For this review, take the finished solid that the model builds, in its own axes (mm). Round coordinates to 2 decimals unless told otherwise and drop trailing zeros. Loops run counter-clockwise (first coordinate to the right, second up) from the corner with the lowest first, then second, coordinate; pieces in that order, holes last. Notation, with made-up numbers: (59.5, 60.25) -> (64.5, 60.25) arc R27 ccw to (64.5, 76.25) -> close; hole circle Ø3 at (87, -17). An arc over 180 degrees is marked (long way). Write each question's results on one line, items separated by ' | '.
```python
from build123d import *

# Parameters (mm, degrees)
SKETCH1_R           = 2.35
BOSS_EXTRUDE1_DEPTH = 7.8


with BuildPart() as part:
    # Sketch1 → Boss-Extrude1 (new body)
    with BuildSketch(Plane(origin=(0, 0, 0), x_dir=(0, 0, -1), z_dir=(1, 0, 0))):
        with BuildLine():
            Line((-56, -3.73), (56, -3.73))
            ThreePointArc((56, -3.73), (59.73, 0), (56, 3.73))
            Line((56, 3.73), (-56, 3.73))
            ThreePointArc((-56, 3.73), (-59.73, 0), (-56, -3.73))
        make_face()
        with Locations((-56, 0)):
            Circle(SKETCH1_R, mode=Mode.SUBTRACT)
        with Locations((-48, 0)):
            Circle(SKETCH1_R, mode=Mode.SUBTRACT)
        with Locations((-40, 0)):
            Circle(SKETCH1_R, mode=Mode.SUBTRACT)
        with Locations((-32, 0)):
            Circle(SKETCH1_R, mode=Mode.SUBTRACT)
        with Locations((-24, 0)):
            Circle(SKETCH1_R, mode=Mode.SUBTRACT)
        with Locations((-16, 0)):
            Circle(SKETCH1_R, mode=Mode.SUBTRACT)
        with Locations((-8, 0)):
            Circle(SKETCH1_R, mode=Mode.SUBTRACT)
        Circle(SKETCH1_R, mode=Mode.SUBTRACT)
        with Locations((8, 0)):
            Circle(SKETCH1_R, mode=Mode.SUBTRACT)
        with Locations((16, 0)):
            Circle(SKETCH1_R, mode=Mode.SUBTRACT)
        with Locations((24, 0)):
            Circle(SKETCH1_R, mode=Mode.SUBTRACT)
        with Locations((32, 0)):
            Circle(SKETCH1_R, mode=Mode.SUBTRACT)
        with Locations((40, 0)):
            Circle(SKETCH1_R, mode=Mode.SUBTRACT)
        with Locations((48, 0)):
            Circle(SKETCH1_R, mode=Mode.SUBTRACT)
        with Locations((56, 0)):
            Circle(SKETCH1_R, mode=Mode.SUBTRACT)
    extrude(amount=BOSS_EXTRUDE1_DEPTH)


solid = part.part
```
1. To check wall thickness, follow probe 1 along Y at (x, z) = (5.5, -40); probe 2 along Y at (x, z) = (0.75, 30); probe 3 along Z at (x, y) = (7, 2.5). State the ranges of each line that lie inside material, in increasing order.
Values found:
probe 1: y = -3.73 to -2.35, 2.35 to 3.73 | probe 2: y = -3.73 to -1.23, 1.23 to 3.73 | probe 3: z = -58.77 to 58.77
2. Draft analysis for pull direction Z (two halves, no side actions). For faces 1 (the face through (3.845, 0.103, 18.348)), 2 (the face through (3.85, -0.08, -59.73)), 3 (the face through (4, 3.73, -1)), state which applies: released by +Z, released by -Z, zero draft, split by the parting line, or undercut.
Values found:
face 1: undercut | face 2: released by -Z | face 3: zero draft
3. For pin 1 (4 mm diameter, centred on y = 0, z = -8, fed in from -X); pin 2 (1.5 mm diameter, centred on y = 0.5, z = 11.5, fed in from -X), all flat-tipped, find the tip position at first contact; note any pin that passes through.
Values found:
pin 1: passes through | pin 2: stops at x = 0
4. Consider section A-A (z = -8). State the section outline as (x, y) points.
Values found:
outline: (0, -3.73) -> (7.8, -3.73) -> (7.8, -2.35) -> (0, -2.35) -> close; (0, 2.35) -> (7.8, 2.35) -> (7.8, 3.73) -> (0, 3.73) -> close
5. Consider section B-B (x = 2). Give the number of separate pieces and of enclosed holes in the cut face, plus the area to 3 significant figures.
Values found:
separate pieces: 1 | enclosed holes: 15 | area: 619 mm2
